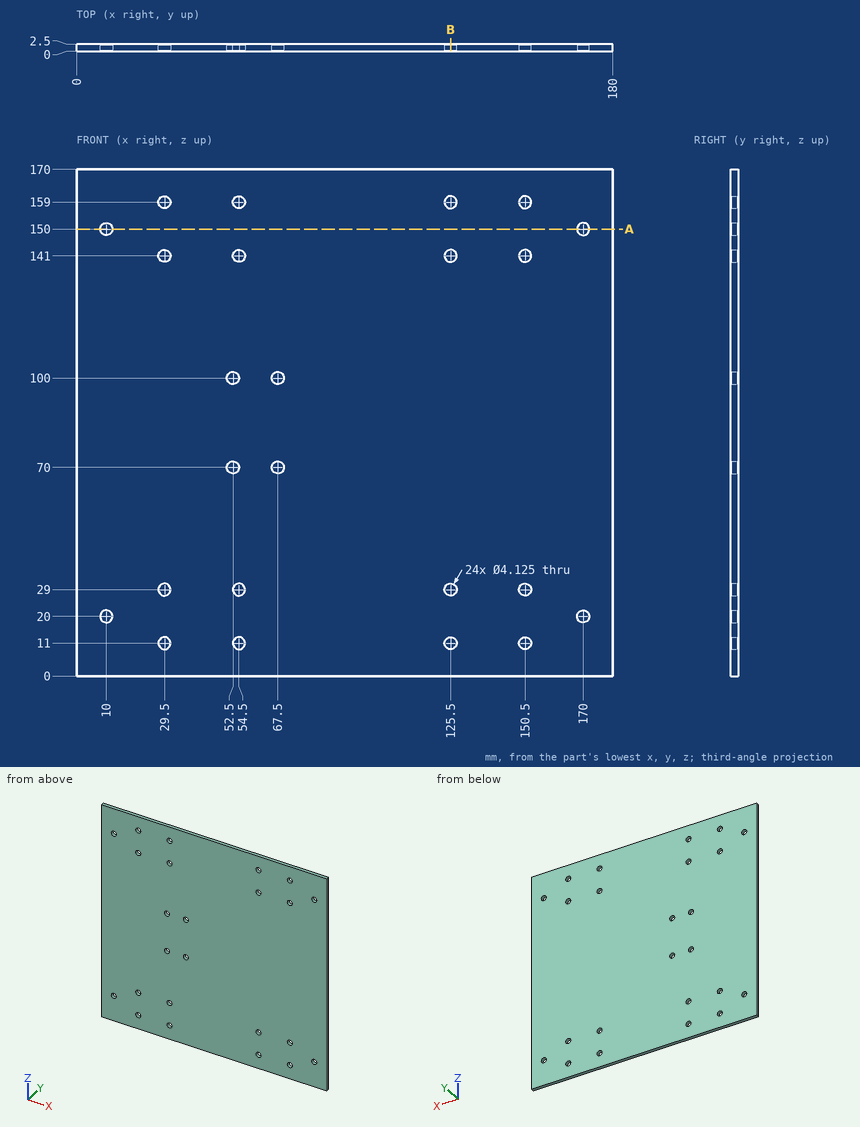
Answer from the drawing. Dimensions are ordinates in mm from the lowest x, y and z of the part. Round coordinates to 2 decimals unless told otherwise and drop trailing zeros. Write each loop counter-clockwise with the first axis right and the second up, starting at its lowest first coordinate (ties: lowest second). Pieces come first, ordered by that corner, then holes. Notation, with made-up numbers: M -30,0 L 17,0 A13 cw 17,20 Z; hole C 41,72 d1. An arc over 180 degrees is marked long. Write each question's results on one line, items separated by ' | '. Start each with the question number.
Item 1: Find section B-B on x = 125.5. Write down the section's boundary in (y, z), and give its area (3 significant figures).
Item 2: Given pin 1 Ø1 at (y, z) = (1.5, 128) entering from -X, flat-ended and moving along its own axis, determine where the tip first touches the part or whether it passes through.
Item 3: Straight lines are drawn through the part: probe 1 along X at (y, z) = (1.5, 150); probe 2 along Z at (x, y) = (150.5, 0.85); probe 3 along Z at (x, y) = (67.5, 1.9). For each, find the intervals that lie inside material, in ascending order.
Item 4: Find section A-A on z = 150. Write down the section's boundary in (x, y), and give its area (3 significant figures).
Answer block:
1) outline: M 0,0 L 2.5,0 L 2.5,8.94 L 0,8.94 Z; M 0,13.06 L 2.5,13.06 L 2.5,26.94 L 0,26.94 Z; M 0,31.06 L 2.5,31.06 L 2.5,138.94 L 0,138.94 Z; M 0,143.06 L 2.5,143.06 L 2.5,156.94 L 0,156.94 Z; M 0,161.06 L 2.5,161.06 L 2.5,170 L 0,170 Z | area: 384 mm²
2) pin 1: stops at x = 0
3) probe 1: x = 0 to 7.94, 12.06 to 167.94, 172.06 to 180 | probe 2: z = 0 to 8.94, 13.06 to 26.94, 31.06 to 138.94, 143.06 to 156.94, 161.06 to 170 | probe 3: z = 0 to 67.94, 72.06 to 97.94, 102.06 to 170
4) outline: M 0,0 L 7.94,0 L 7.94,2.5 L 0,2.5 Z; M 12.06,0 L 167.94,0 L 167.94,2.5 L 12.06,2.5 Z; M 172.06,0 L 180,0 L 180,2.5 L 172.06,2.5 Z | area: 429 mm²
